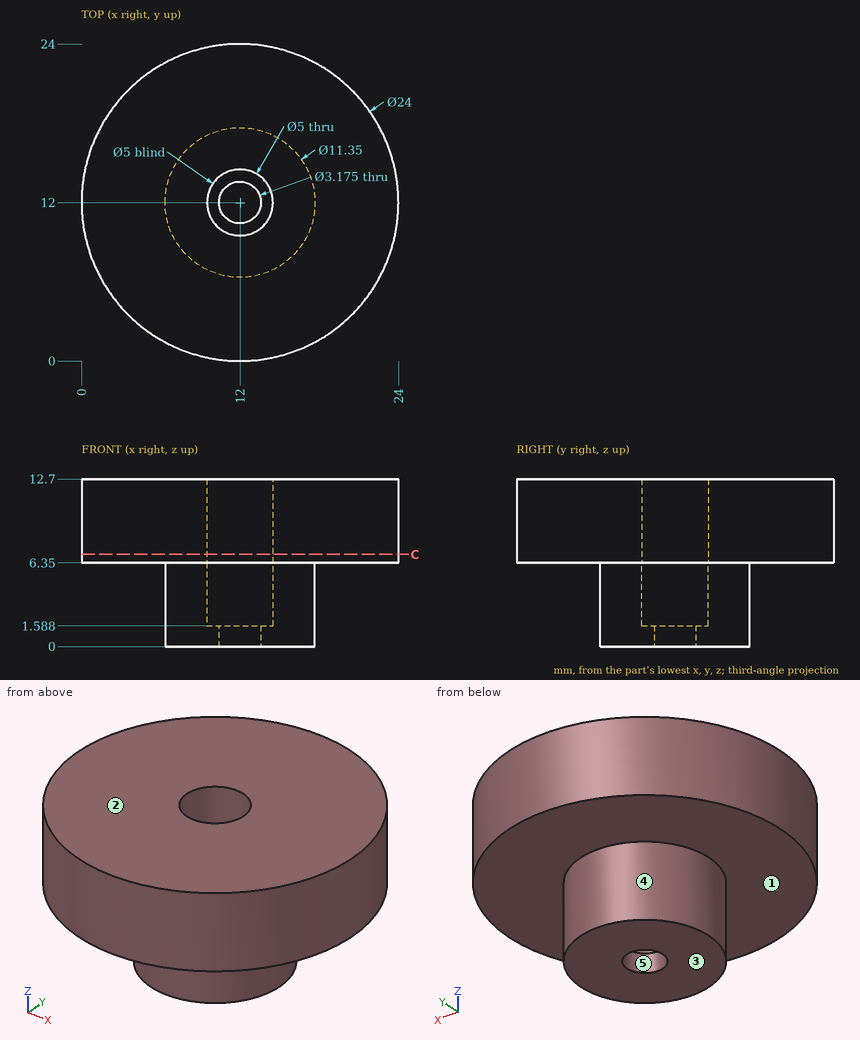
The figure shows three views and two pictorial views of one solid part (mm, origin at its lowest corner). Answer the questions. A direction names the side the tool comes from. Coordinates: 2 decimals unless noted, no trailing zeros. Write each loop counter-clockwise with the first axis right and the second up, starting at its lowest first coordinate (ties: lowest second). Pieces come first, ordered by that corner, then holes. Notation, with made-up numbers: M 15,17 L 42,17 A18 cw 42,41 Z; hole C 2,70.25 d1. An arc over 180 degrees is marked long. Answer as CSV lines item,"result". Start each with the question number.
Item 1: A tool of negligible diameter and unlimited length cuts with its end or side. For the marked faces 1 and 2, from which of +Z, -Z, +X, -X, +Y, -Y can it reach the whole face along a straight path? Write none if from no direction.
Item 2: Flat-ended cylindrical pins translate along their axes: P1, Ø4, axis at x = 10.5, z = 3, coming from the -Y side (1 decimal); P2, Ø4, axis at y = 8.5, z = 11.5, coming from the +X side; P3, Ø1.5, axis at y = 11, z = 4.5, coming from the -X side. Find the tip coordinate at first contact, or state that the pin passes through.
Item 3: Section C-C on z = 7 is taken. Write down the section's boundary in (x, y), and give its area (3 significant figures).
Item 4: Consider L1, parallel to Y at x = 12, z = 4.7 (1 decimal); L2, parallel to Z at x = 20.75, y = 9.5; L3, parallel to Y at x = 12, z = 0.3 (1 decimal). Determine where each line is inside the solid, lowest interval first.
Item 5: Determine the mould class of the marked faces 3, 4 and 5 for opening direction Y: released by +Y, released by -Y, zero draft, split by the parting line, or undercut.
Checks:
1,face 1,"-Z"
1,face 2,"+Z, +X, -X, +Y, -Y"
2,P1,"stops at y = 6.3"
2,P2,"stops at x = 23.91"
2,P3,"stops at x = 6.33"
3,outline,"C 12,12 d24; hole C 12,12 d5"
3,area,"433 mm²"
4,L1,"y = 6.3 to 9.5, 14.5 to 17.7"
4,L2,"z = 6.35 to 12.7"
4,L3,"y = 6.3 to 10.4, 13.6 to 17.7"
5,face 3,"zero draft"
5,face 4,"split by the parting line"
5,face 5,"undercut"
